Autodesk Fusion 360 part; units mm, degrees
sketch "Boceto1" plane through (0, 0, 0) normal (0, 1, 0) x (1, 0, 0)
  line L0 (58, 0) -> (62, 0)
  line L1 (62, 0) -> (62, -4)
  line L2 (62, -4) -> (58, -4)
  line L3 (58, -4) -> (58, 0)
  line L4 (58, -8) -> (62, -8)
  line L5 (62, -8) -> (62, -12)
  line L6 (62, -12) -> (58, -12)
  line L7 (58, -12) -> (58, -8)
  line L8 (62, -12) -> (62, -21)
  line L9 (62, -21) -> (-4, -21)
  line L10 (62, 0) -> (65, 0)
  line L11 (65, 0) -> (65, -24)
  line L12 (65, -24) -> (-7, -24)
  line L13 (29, -21) -> (29, -3)
  line L14 (-4, -12) -> (0, -12)
  line L15 (0, -8) -> (-4, -8)
  line L16 (-4, -8) -> (-4, -12)
  line L17 (-4, -12) -> (-4, -21)
  line L18 (-4, -4) -> (0, -4)
  line L19 (-4, 0) -> (-4, -4)
  line L20 (-4, 0) -> (-7, 0)
  line L21 (-7, 0) -> (-7, -24)
  line L22 (-7, -24) -> (65, -24)
  line L23 (-4, -21) -> (62, -21)
  line L24 (0, 0) -> (-4, 0)
  line L25 (-4, -4) -> (-4, -8)
  line L26 (62, -8) -> (62, -4)
  line L27 (0, -16) -> (0, -8)
  line L28 (0, -4) -> (0, 0)
  line L29 (58, 0) -> (58, -4)
  line L30 (58, -8) -> (58, -16)
  dimension "d1" = 58
  dimension "d2" = 16
  dimension "d3" = 4
  dimension "d4" = 4
  dimension "d5" = 4
  dimension "d6" = 4
  dimension "d7" = 4
  dimension "d8" = 9
  dimension "d9" = 66
  dimension "d10" = 24
  dimension "d11" = 72
extrude "Extruir1" add sketch "Boceto1" along normal blind 100
sketch "Boceto2" plane through (0, 100, 0) normal (0, 1, 0) x (-1, 0, 0)
  line L0 (-62, 8) -> (-58, 8)
  line L1 (-58, 8) -> (-58, 12)
  line L2 (-58, 12) -> (-62, 12)
  line L3 (-62, 12) -> (-62, 21)
  line L4 (-62, 21) -> (4, 21)
  line L5 (4, 21) -> (4, 12)
  line L6 (4, 12) -> (0, 12)
  line L7 (0, 12) -> (0, 8)
  line L8 (0, 8) -> (4, 8)
  line L9 (4, 8) -> (4, 4)
  line L10 (4, 4) -> (0, 4)
  line L11 (0, 4) -> (0, 0)
  line L12 (0, 0) -> (7, 0)
  line L13 (7, 0) -> (7, 24)
  line L14 (7, 24) -> (-65, 24)
  line L15 (-65, 24) -> (-65, 0)
  line L16 (-65, 0) -> (-58, 0)
  line L17 (-58, 0) -> (-58, 4)
  line L18 (-58, 4) -> (-62, 4)
  line L19 (-62, 4) -> (-62, 8)
  line L20 (7, 0) -> (-65, 0)
  line L21 (-65, 0) -> (-65, 24)
  line L22 (-65, 24) -> (7, 24)
  line L23 (7, 24) -> (7, 0)
extrude "Extruir2" add sketch "Boceto2" against normal blind 3 contours L0 L1 L2 L3 L4 L5 L6 L7 L8 L9 L10 L11 L17 L18 L19 L20
move_face "CarasDesfase1" offset -0.2 14 faces at (58, 32.3333, 2.6667) (58, 32.3333, 10.6667) (62, 32.3333, 15) (59.3333, 32.3333, 8) (62, 32.3333, 6.6667) (0, 32.3333, 2.6667) (-4, 32.3333, 5.3333) (0, 32.3333, 10.6667) (-4, 32.3333, 15) (-1.3333, 32.3333, 8) (-2.6667, 32.3333, 4) (-2.6667, 32.3333, 12) (59.3333, 64.6667, 4) (59.3333, 64.6667, 12)
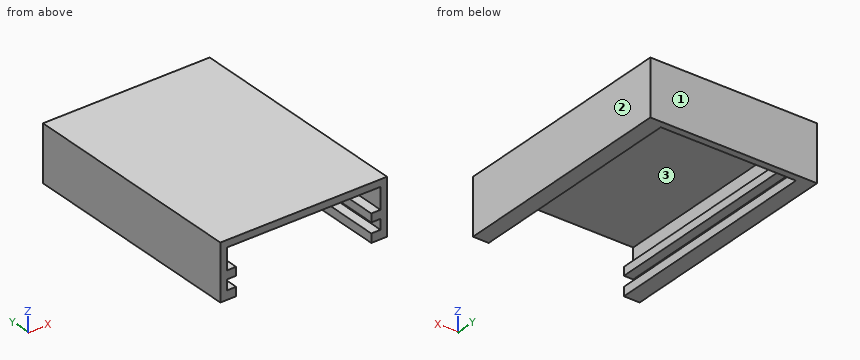
Design review of the part built by this model. Coordinates are the model's own, in mm. Face numbers are marked on the shaded views. Round coordinates to 2 decimals unless told otherwise and drop trailing zeros. Write each loop counter-clockwise with the first axis right and the second up, starting at its lowest first coordinate (ties: lowest second). Pieces come first, ordered by that corner, then holes. Notation, with made-up numbers: (-26, 64) -> (32, 64) arc R19 ccw to (32, 85) -> close; hole circle Ø10 at (48.25, 31.5). An arc over 180 degrees is marked (long way). One line per item, written item: value. Start each with the question number.
Q1. Add section C-C (x = 11). Give the boundary of the cut face in (y, z).
Q2. Insertion check: P1, Ø10, axis at x = 36, y = 56.5, coming from the -Z side; P2, Ø8, axis at x = 53, z = 3, coming from the -Y side. Each pin has a flat end and moves straight along its axis. Give the tip position at first contact, or say it passes through.
Q3. Add section A-A (y = 26). Give the boundary of the cut face in (x, z), then the cut area to 3 significant figures.
Q4. Add section B-B (z = 19.25). Give the boundary of the cut face in (x, y), then the cut area to 3 significant figures.
Q5. Add section D-D (z = 1.5). Give the boundary of the cut face in (x, y).
Q6. To check wall thickness, follow probe 1 along Z at (x, y) = (61.5, 6.5); probe 2 along X at (y, z) = (34, 14.25); probe 3 along X at (y, z) = (93, 2.5). State the ranges of each line that lie inside material, in increasing order.
Q7. The part is to be moulded in two halves that separate along X. For the marked faces 1, 2 and 3, say which applies: pulls with the +X half, pulls with the -X half, needs draft (parallel to the pull), parting line crosses it, or undercut.
Response:
1. outline: (0, 21) -> (97, 21) -> (97, 0) -> (100, 0) -> (100, 24) -> (0, 24) -> close
2. P1: stops at z = 21
2. P2: stops at y = 97
3. outline: (-7, 0) -> (-0.2, 0) -> (-0.2, 3.8) -> (-4.2, 3.8) -> (-4.2, 8.2) -> (-0.2, 8.2) -> (-0.2, 11.8) -> (-4.2, 11.8) -> (-4.2, 21) -> (62.2, 21) -> (62.2, 11.8) -> (58.2, 11.8) -> (58.2, 8.2) -> (62.2, 8.2) -> (62.2, 3.8) -> (58.2, 3.8) -> (58.2, 0) -> (65, 0) -> (65, 24) -> (-7, 24) -> close
3. area: 393 mm^2
4. outline: (-7, 0) -> (-4.2, 0) -> (-4.2, 97) -> (62.2, 97) -> (62.2, 0) -> (65, 0) -> (65, 100) -> (-7, 100) -> close
4. area: 759 mm^2
5. outline: (-7, 0) -> (-0.2, 0) -> (-0.2, 97) -> (58.2, 97) -> (58.2, 0) -> (65, 0) -> (65, 100) -> (-7, 100) -> close
6. probe 1: z = 0 to 3.8, 8.2 to 11.8, 21 to 24
6. probe 2: x = -7 to -4.2, 62.2 to 65
6. probe 3: x = -7 to -0.2, 58.2 to 65
7. face 1: needs draft
7. face 2: pulls with the +X half
7. face 3: undercut
